Verification items for the finished model (mm, model axes). Face numbers are marked on the shaded views. A direction names the side the tool comes from. Coordinates: 2 decimals unless noted, no trailing zeros. Write each loop counter-clockwise with the first axis right and the second up, starting at its lowest first coordinate (ties: lowest second). Pieces come first, ordered by that corner, then holes. Notation, with made-up numbers: (89.25, 11.25) -> (119.25, 11.25) arc R22 cw to (119.25, 28.25) -> close; hole circle Ø10 at (61, 59.25). An arc over 180 degrees is marked (long way). Write item = value, one per line. Start each with the question number.
(1) Section check A-A (x = 27). Record the cut outline in (y, z).
(2) Mould release check, pull along Y, two halves, no side actions. Record for the marked faces 3, 4 and 5: released by +Y, released by -Y, zero draft, split by the parting line, or undercut.
(3) Section check D-D (x = 31.5). Record the cut outline in (y, z).
(4) Section check B-B (z = 5). State how many separate pieces and enclosed holes the cut face has, plus the area to 3 significant figures.
(5) Gauge pin test, flat ends, axial feed: pin 1 Ø1 at (y, z) = (38, 4.5) entering from +X; pin 2 Ø14.5 at (x, y) = (14, 25) entering from +Z. Record the tip position at first contact, or that the pin passes through.
(6) Material ranges on probe 1 along Y at (x, z) = (23.5, 5); probe 2 along Y at (x, z) = (17, 1.05); probe 3 along Y at (x, z) = (17, 2.1), recorded low to high. Write a range as [from, to].
(7) Section check C-C (y = 35.6). Record the cut outline in (x, z).
(8) Set-up check for the marked faces 1 and 2: record each of +Z, -Z, +X, -X, +Y, -Y from which the full face is reachable in a straight line by a thin tool's end or side.
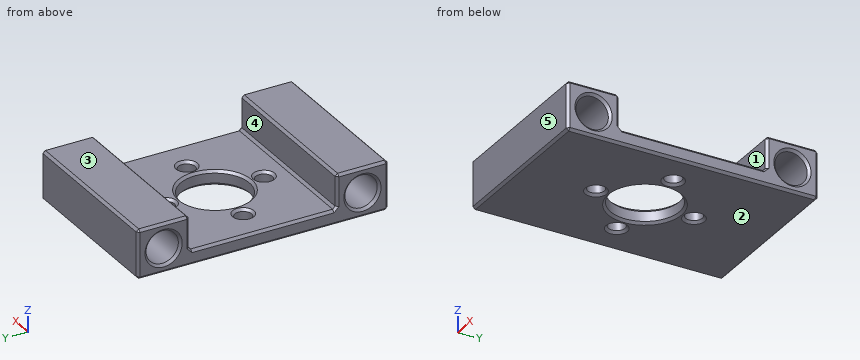
```python
from build123d import *

# Parameters (mm, degrees)
ESQUISSE1_W             = 34
ESQUISSE1_H             = 51.2
BOSS_EXTRU_1_DEPTH      = 10
ESQUISSE4_W             = 34
ESQUISSE4_H             = 30
ENL_V_MAT_EXTRU_1_DEPTH = 7
ESQUISSE5_R             = 7
ENL_V_MAT_EXTRU_2_DEPTH = 62.858224999
D_GAGEMENT_M62_D        = 6.6
D_GAGEMENT_M31_D        = 3.4
CHANFREIN1_SIZE         = 0.5


with BuildPart() as part:
    # Esquisse1 → Boss.-Extru.1 (new body)
    with BuildSketch(Plane.XY):
        with Locations((17, 25.6)):
            Rectangle(ESQUISSE1_W, ESQUISSE1_H)
    extrude(amount=BOSS_EXTRU_1_DEPTH)

    # Esquisse4 → Enlèv. mat.-Extru.1 (cut)
    with BuildSketch(Plane.XY.offset(10)):
        with Locations((17, 25.6)):
            Rectangle(ESQUISSE4_W, ESQUISSE4_H)
    extrude(amount=-ENL_V_MAT_EXTRU_1_DEPTH, mode=Mode.SUBTRACT)

    # Esquisse5 → Enlèv. mat.-Extru.2 (cut, through all)
    with BuildSketch(Plane.XY.offset(3)):
        with Locations((17, 25.6)):
            Circle(ESQUISSE5_R)
    extrude(amount=-ENL_V_MAT_EXTRU_2_DEPTH, mode=Mode.SUBTRACT)

    # Dégagement M62 (through all)
    with Locations(Plane.ZY):
        with Locations((5, 45.9), (5, 5.3)):
            Hole(D_GAGEMENT_M62_D / 2)

    # Dégagement M31 (through all)
    with Locations(Plane.XY.offset(3)):
        with Locations((17, 35.6), (7, 25.6), (17, 15.6), (27, 25.6)):
            Hole(D_GAGEMENT_M31_D / 2)

    # Chanfrein1
    chanfrein1_edges = [part.edges().sort_by_distance(p)[0] for p in [
        (34, 5.3, 10),
        (17, 51.2, 10),
        (0, 5.3, 10),
        (34, 45.9, 10),
        (0, 25.6, 3),
        (0, 10.6, 6.5),
        (17, 40.6, 3),
        (0, 40.6, 6.5),
        (34, 25.6, 3),
        (34, 40.6, 6.5),
        (17, 10.6, 3),
        (34, 10.6, 6.5),
        (17, 10.6, 10),
        (17, 40.6, 10),
        (10, 25.6, 0),
        (10, 25.6, 3),
        (0, 5.3, 8.3),
        (34, 5.3, 8.3),
        (0, 45.9, 10),
        (0, 45.9, 8.3),
        (34, 45.9, 8.3),
        (17, 51.2, 0),
        (34, 25.6, 0),
        (28.7, 25.6, 3),
        (28.7, 25.6, 0),
        (17, 0, 0),
        (18.7, 15.6, 3),
        (18.7, 15.6, 0),
        (0, 25.6, 0),
        (8.7, 25.6, 3),
        (8.7, 25.6, 0),
        (18.7, 35.6, 3),
        (18.7, 35.6, 0),
        (17, 0, 10),
        (0, 51.2, 5),
        (34, 51.2, 5),
        (34, 0, 5),
        (0, 0, 5),
    ]]
    chamfer(chanfrein1_edges, length=CHANFREIN1_SIZE)


solid = part.part
```
Response:
q1.outline = (0, 0.5) -> (0.5, 0) -> (23.4, 0) -> (23.9, 0.5) -> (23.9, 2.5) -> (23.4, 3) -> (11.1, 3) -> (10.6, 3.5) -> (10.6, 9.5) -> (10.1, 10) -> (0.5, 10) -> (0, 9.5) -> close; (27.3, 0.5) -> (27.8, 0) -> (50.7, 0) -> (51.2, 0.5) -> (51.2, 9.5) -> (50.7, 10) -> (41.1, 10) -> (40.6, 9.5) -> (40.6, 3.5) -> (40.1, 3) -> (27.8, 3) -> (27.3, 2.5) -> close; hole circle Ø6.6 at (5.3, 5); hole circle Ø6.6 at (45.9, 5)
q2.face_3 = zero draft
q2.face_4 = undercut
q2.face_5 = released by -Y
q3.outline = (0, 0.5) -> (0.5, 0) -> (50.7, 0) -> (51.2, 0.5) -> (51.2, 9.5) -> (50.7, 10) -> (41.1, 10) -> (40.6, 9.5) -> (40.6, 3.5) -> (40.1, 3) -> (11.1, 3) -> (10.6, 3.5) -> (10.6, 9.5) -> (10.1, 10) -> (0.5, 10) -> (0, 9.5) -> close; hole circle Ø6.6 at (5.3, 5); hole circle Ø6.6 at (45.9, 5)
q4.separate_pieces = 4
q4.enclosed_holes = 0
q4.area = 270 mm2
q5.pin_1 = through
q5.pin_2 = 3
q6.probe_1 = [0, 2], [8.6, 10.6], [40.6, 42.6], [49.2, 51.2]
q6.probe_2 = [0, 13.9], [17.3, 18.6], [32.6, 33.9], [37.3, 51.2]
q6.probe_3 = [0, 3.73], [6.87, 13.9], [17.3, 18.6], [32.6, 33.9], [37.3, 44.33], [47.47, 51.2]
q7.outline = (0, 0.5) -> (0.5, 0) -> (14.8, 0) -> (15.3, 0.5) -> (15.3, 2.5) -> (14.8, 3) -> (0.5, 3) -> (0, 2.5) -> close; (18.7, 0.5) -> (19.2, 0) -> (33.5, 0) -> (34, 0.5) -> (34, 2.5) -> (33.5, 3) -> (19.2, 3) -> (18.7, 2.5) -> close
q8.face_1 = +Z, +X, -X
q8.face_2 = -Z, +X, -X, +Y, -Y
